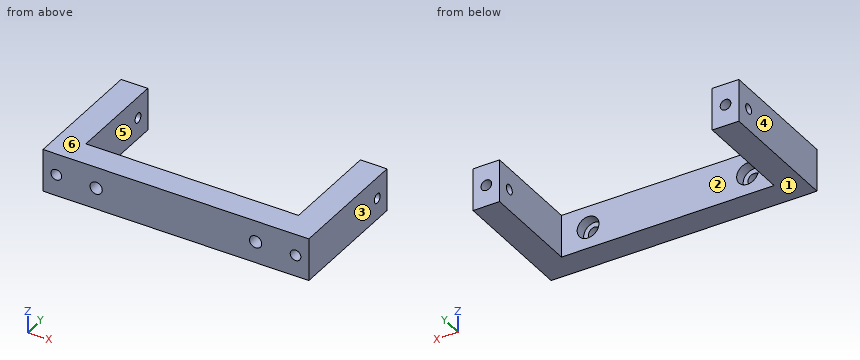
from build123d import *

# Parameters (mm, degrees)
SKETCH1_W           = 50
SKETCH1_H           = 8
BOSS_EXTRUDE1_DEPTH = 5
SKETCH5_W           = 8
SKETCH5_H           = 24
SKETCH5_R           = 0.9
BOSS_EXTRUDE3_DEPTH = 5
CUT_EXTRUDE3_REACH  = 36.886
SKETCH6_R           = 1
SKETCH2_R           = 1.15
CUT_EXTRUDE1_DEPTH  = 35.885527225
CUT_EXTRUDE4_REACH  = 39.886
CUT_EXTRUDE4_START  = -3
SKETCH7_R           = 2.05


with BuildPart() as part:
    # Sketch1 → Boss-Extrude1 (new body)
    with BuildSketch(Plane(origin=(0, 0, 0), x_dir=(1, 0, 0), z_dir=(0, 1, 0))):
        Rectangle(SKETCH1_W, SKETCH1_H)
    extrude(amount=BOSS_EXTRUDE1_DEPTH)

    # Sketch5 → Boss-Extrude3 (add)
    with BuildSketch(Plane(origin=(25, 0, 0), x_dir=(0, 0, -1), z_dir=(1, 0, 0))):
        with Locations((0, 12)):
            Rectangle(SKETCH5_W, SKETCH5_H)
        with Locations((0, 21)):
            Circle(SKETCH5_R, mode=Mode.SUBTRACT)
    boss_extrude3 = extrude(amount=-BOSS_EXTRUDE3_DEPTH)

    # Sketch6 → Cut-Extrude3 (cut, up to next)
    with BuildSketch(Plane(origin=(0, 24, 0), x_dir=(1, 0, 0), z_dir=(0, 1, 0)), mode=Mode.PRIVATE) as cut_extrude3_sk1:
        with Locations(Location((22.5, 0, 0), (0, 0, 270))):
            Circle(SKETCH6_R)
    cut_extrude3_tool1 = extrude(cut_extrude3_sk1.sketch, amount=-CUT_EXTRUDE3_REACH, mode=Mode.PRIVATE) & part.part
    cut_extrude3 = cut_extrude3_tool1.solids().sort_by_distance((22.5, 24, 0))[0]
    add(cut_extrude3, mode=Mode.SUBTRACT)

    # Sketch2 → Cut-Extrude1 (cut, through all)
    with BuildSketch(Plane(origin=(0, 0, 0), x_dir=(1, 0, 0), z_dir=(0, 1, 0))):
        with Locations(Location((15, 0, 0), (0, 0, 90))):
            Circle(SKETCH2_R)
    cut_extrude1 = extrude(amount=CUT_EXTRUDE1_DEPTH, mode=Mode.SUBTRACT)

    # Sketch7 → Cut-Extrude4 (cut, up to next)
    with BuildSketch(Plane.XZ.offset(CUT_EXTRUDE4_START), mode=Mode.PRIVATE) as cut_extrude4_sk1:
        with Locations(Location((15, 0, 0), (0, 0, 270))):
            Circle(SKETCH7_R)
    cut_extrude4_tool1 = extrude(cut_extrude4_sk1.sketch, amount=-CUT_EXTRUDE4_REACH, mode=Mode.PRIVATE) & part.part
    cut_extrude4 = cut_extrude4_tool1.solids().sort_by_distance((15, 3, 0))[0]
    add(cut_extrude4, mode=Mode.SUBTRACT)

    # Mirror5: Boss-Extrude3, Cut-Extrude3, Cut-Extrude1, Cut-Extrude4 across plane
    add(boss_extrude3.mirror(Plane(origin=(0, 0, 0), x_dir=(0, 0, 1), z_dir=(1, 0, 0))))
    add(cut_extrude3.mirror(Plane(origin=(0, 0, 0), x_dir=(0, 0, 1), z_dir=(1, 0, 0))), mode=Mode.SUBTRACT)
    add(cut_extrude1.mirror(Plane(origin=(0, 0, 0), x_dir=(0, 0, 1), z_dir=(1, 0, 0))), mode=Mode.SUBTRACT)
    add(cut_extrude4.mirror(Plane(origin=(0, 0, 0), x_dir=(0, 0, 1), z_dir=(1, 0, 0))), mode=Mode.SUBTRACT)


solid = part.part
Source: CAD feature listing. Evaluate the final solid. Frame: model axes, mm. Face numbers are marked on the shaded views. A direction names the side the tool comes from. Give positions to 0.01 mm unless a question says otherwise; leave off trailing zeros. Write each loop counter-clockwise with the first axis right and the second up, starting at its lowest first coordinate (ties: lowest second). Pieces come first, ordered by that corner, then holes. Notation, with made-up numbers: (84, -24) -> (126, -24) arc R16 cw to (126, -13) -> close; hole circle Ø9 at (45, 54.25). An arc over 180 degrees is marked (long way). Return JSON: item names as keys, results as strings. Group by question number.
1. Section C-C, the plane y = 21. Output: boundary loops of the cut face in (x, z).
2. Access query for the marked faces 5 and 6. Directions: +Z, -Z, +X, -X, +Y, -Y. A direction counts if a zero-diameter tool reaches every point of the face in a straight line with its end or side. Return the directions, or none.
3. Section B-B, the plane x = -15. Output: boundary loops of the cut face in (y, z), then the cut area to 3 significant figures.
4. Material intervals for line 1 (X direction, y = 9.5, z = 0); line 2 (X direction, y = 12.25, z = -1.25); line 3 (X direction, y = 9, z = -0.5), sorted ascending. Write a range as from..to.
5. Section A-A, the plane y = 5.75. Output: boundary loops of the cut face in (x, z).
6. Mould query, pull axis X, two halves, no side actions, for the marked faces 1, 2, 3 and 4. Classes: +X half, -X half, draft (parallel to the pull), parting line (faces both ways), or undercut.
7. Section D-D, the plane z = -2.75. Output: boundary loops of the cut face in (x, y).
8. Pin query (flat end, axial travel): pin 1 Ø1.6 at (y, z) = (21, 0) entering from +X; pin 2 Ø4 at (x, z) = (7, -2) entering from +Y; pin 3 Ø4 at (x, y) = (-19, 16.5) entering from -Z; pin 4 Ø1.2 at (x, z) = (16, 1) entering from +Y. Return the tip coordinate at first contact, or that it passes through.
Determined:
{
 "1": {"outline": "(-25, -4) -> (-20, -4) -> (-20, -0.9) -> (-22.06, -0.9) arc R1 cw to (-22.94, -0.9) -> (-25, -0.9) -> close; (-25, 0.9) -> (-22.94, 0.9) arc R1 cw to (-22.06, 0.9) -> (-20, 0.9) -> (-20, 4) -> (-25, 4) -> close; (20, -4) -> (25, -4) -> (25, -0.9) -> (22.94, -0.9) arc R1 cw to (22.06, -0.9) -> (20, -0.9) -> close; (20, 0.9) -> (22.06, 0.9) arc R1 cw to (22.94, 0.9) -> (25, 0.9) -> (25, 4) -> (20, 4) -> close"},
 "2": {"face 5": "+Z, -Z, +Y", "face 6": "+Z, +X, -X, +Y, -Y"},
 "3": {"outline": "(0, -4) -> (5, -4) -> (5, -2.05) -> (3, -2.05) -> (3, -1.15) -> (0, -1.15) -> close; (0, 1.15) -> (3, 1.15) -> (3, 2.05) -> (5, 2.05) -> (5, 4) -> (0, 4) -> close", "area": "24.9 mm2"},
 "4": {"line 1": "x = -25..-23.5, -21.5..-20, 20..21.5, 23.5..25", "line 2": "x = -25..-20, 20..25", "line 3": "x = -25..-23.37, -21.63..-20, 20..21.63, 23.37..25"},
 "5": {"outline": "(-25, -4) -> (-20, -4) -> (-20, 4) -> (-25, 4) -> close; (20, -4) -> (25, -4) -> (25, 4) -> (20, 4) -> close; hole circle Ø2 at (-22.5, 0); hole circle Ø2 at (22.5, 0)"},
 "6": {"face 1": "draft", "face 2": "undercut", "face 3": "+X half", "face 4": "-X half"},
 "7": {"outline": "(-25, 0) -> (25, 0) -> (25, 24) -> (20, 24) -> (20, 5) -> (-20, 5) -> (-20, 24) -> (-25, 24) -> close"},
 "8": {"pin 1": "passes through", "pin 2": "stops at y = 5", "pin 3": "stops at z = -4", "pin 4": "stops at y = 3"}
}
